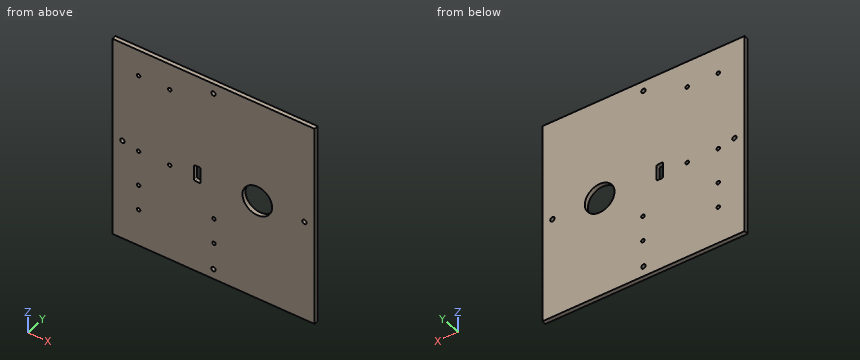
```python
from build123d import *

# Parameters (mm, degrees)
SKETCH1_W           = 150
SKETCH1_H           = 150
SKETCH1_R           = 1.65
SKETCH1_R_2         = 1.3
SKETCH1_R_3         = 11
BOSS_EXTRUDE1_DEPTH = 3.175


with BuildPart() as part:
    # Sketch1 → Boss-Extrude1 (new body)
    with BuildSketch(Plane(origin=(0, 0, 0), x_dir=(1, 0, 0), z_dir=(0, 1, 0))):
        Rectangle(SKETCH1_W, SKETCH1_H)
        with Locations(Location((-67.5, 0, 0), (0, 0, 270))):
            Circle(SKETCH1_R, mode=Mode.SUBTRACT)
        with Locations(Location((0, 67.5, 0), (0, 0, 270))):
            Circle(SKETCH1_R, mode=Mode.SUBTRACT)
        with Locations(Location((67.5, 0, 0), (0, 0, 270))):
            Circle(SKETCH1_R, mode=Mode.SUBTRACT)
        with Locations(Location((0, -67.5, 0), (0, 0, 270))):
            Circle(SKETCH1_R, mode=Mode.SUBTRACT)
        with Locations(Location((-55.5, -55.5, 0), (0, 0, 270))):
            Circle(SKETCH1_R_2, mode=Mode.SUBTRACT)
        with Locations(Location((-32.45, -55.5, 0), (0, 0, 270))):
            Circle(SKETCH1_R_2, mode=Mode.SUBTRACT)
        with Locations(Location((-32.45, 2.55, 0), (0, 0, 270))):
            Circle(SKETCH1_R_2, mode=Mode.SUBTRACT)
        with Locations(Location((-55.5, 2.55, 0), (0, 0, 270))):
            Circle(SKETCH1_R_2, mode=Mode.SUBTRACT)
        with Locations(Location((0.4, 47.5, 0), (0, 0, 270))):
            Circle(SKETCH1_R_2, mode=Mode.SUBTRACT)
        with Locations(Location((0.4, 28.7, 0), (0, 0, 270))):
            Circle(SKETCH1_R_2, mode=Mode.SUBTRACT)
        with Locations(Location((-55.5, 47.5, 0), (0, 0, 270))):
            Circle(SKETCH1_R_2, mode=Mode.SUBTRACT)
        with Locations(Location((-55.5, 28.7, 0), (0, 0, 270))):
            Circle(SKETCH1_R_2, mode=Mode.SUBTRACT)
        with Locations(Location((32.5, 0, 0), (0, 0, 270))):
            Circle(SKETCH1_R_3, mode=Mode.SUBTRACT)
        with BuildLine():
            Line((-13.534289991, -6), (-10.534289991, -6))
            ThreePointArc((-10.534289991, -6), (-9.82718321, -5.707106781), (-9.534289991, -5))
            Line((-9.534289991, -5), (-9.534289991, 5))
            ThreePointArc((-9.534289991, 5), (-9.82718321, 5.707106781), (-10.534289991, 6))
            Line((-10.534289991, 6), (-13.534289991, 6))
            ThreePointArc((-13.534289991, 6), (-14.241396772, 5.707106781), (-14.534289991, 5))
            Line((-14.534289991, 5), (-14.534289991, -5))
            ThreePointArc((-14.534289991, -5), (-14.241396772, -5.707106781), (-13.534289991, -6))
        make_face(mode=Mode.SUBTRACT)
    extrude(amount=BOSS_EXTRUDE1_DEPTH)


solid = part.part
```
Could you check a few things on this model? Use its own coordinates, in mm. Coordinates: 2 decimals unless noted, no trailing zeros. Order: outer loops, then holes, each group sorted by start corner. A loop starts at its lowest first (then second) coordinate and runs counter-clockwise, first axis right, second up. Notation, with made-up numbers: M -16,-19.5 L -10,-19.5 A7 cw -10,-14.5 Z; hole C -22,43.25 d7. An arc over 180 degrees is marked long. Use one line per item in the form item = value. Start each with the question number.
1. Suppose I cut it at C-C on z = -9. Write out the boundary of the cut face in (x, y) (3 decimals), then the cut area to 3 significant figures.
2. Suppose I cut it at B-B on y = 1.3. Count the separate pieces of the cut face and the enclosed holes in it, then the cut area to 3 significant figures.
3. Please list where these lines run through material, in increasing order: line 1 (X direction, y = 0.85, z = 55.5); line 2 (X direction, y = 0.8, z = -28.7); line 3 (Z direction, x = -67.5, y = 0.75).
4. Suppose I cut it at A-A on x = 32.5. Write out the boundary of the cut face in (y, z) (3 decimals), then the cut area to 3 significant figures.
Geometry says:
q1.outline = M -75,0 L 26.175,0 L 26.175,3.175 L -75,3.175 Z; M 38.825,0 L 75,0 L 75,3.175 L 38.825,3.175 Z
q1.area = 436 mm^2
q2.separate_pieces = 1
q2.enclosed_holes = 14
q2.area = 22,000 mm^2
q3.line_1 = -75 to -56.8, -54.2 to -33.75, -31.15 to 75
q3.line_2 = -75 to -56.8, -54.2 to -0.9, 1.7 to 75
q3.line_3 = -75 to -1.65, 1.65 to 75
q4.outline = M 0,-75 L 3.175,-75 L 3.175,-11 L 0,-11 Z; M 0,11 L 3.175,11 L 3.175,75 L 0,75 Z
q4.area = 406 mm^2
